Work out the finished part from the listing and answer in its coordinate system (mm). A direction names the side the tool comes from. Round coordinates to 2 decimals unless told otherwise and drop trailing zeros. Order: outer loops, then holes, each group sorted by start corner. A loop starts at its lowest first (then second) coordinate and runs counter-clockwise, first axis right, second up. Notation, with made-up numbers: M -18.5,20 L 19.5,20 A31 cw 19.5,54 Z; hole C -35.5,73 d7. An arc over 180 degrees is marked long. Answer as a JSON object with one key per item and string values. Group by question number.
Autodesk Inventor part; units mm, degrees
ref_plane "YZ Plane" through (0, 0, 0) normal (1, 0, 0) x (0, 1, 0)
ref_plane "XZ Plane" through (0, 0, 0) normal (0, 1, 0) x (-1, 0, 0)
ref_plane "XY Plane" through (0, 0, 0) normal (0, 0, 1) x (1, 0, 0)
sketch "Sketch1" plane through (0, 0, 0) normal (0, 0, 1) x (1, 0, 0)
  circle A0 centre (0, 0) radius 0.5
  circle A1 centre (0.0161, 0) radius 1.5
  line L0 (-5.3807, 0) -> (21.8968, 0)
  line L1 (0.0161, 0) -> (15.0161, 0)
  line L2 (15.0161, 0) -> (18, 0)
  line L3 (18, 0) -> (0.9161, 1.2)
  line L4 (18, 0) -> (0.9161, -1.2)
  dimension "d0" = 1
  dimension "d1" = 3
  dimension "d3" = 2.4
  dimension "d13" = 18
extrude "Extrusion1" add sketch "Sketch1" along normal blind 1 contours L0 A1 A0 | A0 L0 A1 | L0 L4 A1 | A1 L3 L0
sketch "Sketch2" plane through (0, 0, 0) normal (0, 0, -1) x (-1, 0, 0)
  circle A0 centre (0, 0) radius 0.5
  circle A1 centre (0.0161, 0) radius 1.5
  line L0 (-5.7839, 0) -> (24.3161, 0)
  line L1 (0.0161, 0) -> (20.0161, 0)
  line L2 (20.0161, 0) -> (20.0155, 0)
  line L3 (20.0155, 0) -> (0.8452, 1.25)
  line L4 (20.0155, 0) -> (0.8452, -1.25)
  dimension "d6" = 1
  dimension "d7" = 3
  dimension "d8" = 20
  dimension "d9" = 2.5
extrude "Extrusion2" add sketch "Sketch2" along normal blind 1 contours L0 A1 A0 | A0 L0 A1
equation "\"d0\" = pointer_axis"
equation "\"d1\" = pointer_axis_outside"
equation "\"d3\" = 0.8 * pointer_axis_outside"
equation "\"circle_dimension\" = 56"
equation "\"circle_dimension_inner\" = 47"
equation "\"hole_from_center\" = 63.5"
equation "\"hole_distance\" = 22.45064"
equation "\"ring_depth\" = 6"
equation "\"ring_thickness\" = 9"
equation "\"ring_top_thickness\" = 2"
equation "\"ring_outer_bevel_height\" = 3"
equation "\"ring_outer_bevel_depth\" = 0.5"
equation "\"ring_inner_bevel_depth\" = 3.5"
equation "\"screw_distance_center\" = 15"
equation "\"screw_distance_outside\" = 3.5"
equation "\"front_plate_thickness\" = 2"
equation "\"glass_thickness\" = 2"
equation "\"encoders\" = 0"
equation "\"encoder_axis\" = 8"
equation "\"encoder_emboss\" = 0"
equation "\"encoder_width\" = 27"
equation "\"encoder_rad\" = 49"
equation "\"encoder_extrude_hight\" = 3"
equation "\"pointer_axis\" = 1"
equation "\"pointer_axis_outside\" = 3"
equation "\"pointer_length\" = 18"
properties part number "pointer_small" material "ABS Plastic"
Item 1: Find section A-A (z = -0.8). Give the vertices of the cut face in (x, y).
Item 2: Find section C-C (x = 8). Give the vertices of the cut face in (y, z), and give its area (3 significant figures).
Item 3: A tool of negligible diameter and unlimited length cuts with its end or side. For faces 1 (the cylindrical face through (1.174, 0.913, -0.493)), 2 (the flat face through (-1, 0, -1)), 3 (the cylindrical face through (-1.483, -0.046, 0.493)), from which of +Z, -Z, +X, -X, +Y, -Y can it reach the whole face along a straight path? Write none if from no direction.
Item 4: Find section D-D (z = 0.75). Give the vertices of the cut face in (x, y), and give its area (3 significant figures).
Item 5: Consider L1, parallel to X at y = 0, z = -0.45; L2, parallel to Y at x = 0, z = -0.65; L3, parallel to Z at x = 10.5, y = 0.25. Determine where each line is inside the solid, lowest interval first.
Responses:
{
 "1": {"outline": "C -0.02,0 d3; hole C 0,0 d1"},
 "2": {"outline": "M -0.7,0 L 0.7,0 L 0.7,1 L -0.7,1 Z", "area": "1.40 mm^2"},
 "3": {"face 1": "-Z", "face 2": "-Z, +X, -X, +Y, -Y", "face 3": "+Z"},
 "4": {"outline": "M 0.92,-1.2 L 18,0 L 0.92,1.2 A1.5 ccw long Z; hole C 0,0 d1", "area": "25.8 mm^2"},
 "5": {"L1": "x = -1.52 to -0.5, 0.5 to 1.48", "L2": "y = -1.5 to -0.5, 0.5 to 1.5", "L3": "z = 0 to 1"}
}
